Geometry check sheet. Reference: the model listing, model coordinates, mm. A direction names the side the tool comes from. Coordinates: 2 decimals unless noted, no trailing zeros. Loops run counter-clockwise (first coordinate to the right, second up) from the corner with the lowest first, then second, coordinate; pieces in that order, holes last.
from build123d import *

# Parameters (mm, degrees)
F1_DEPTH    = 10
F2_T1_DEPTH = 36.6968120455
F3_W        = 4.5079379342
F3_H        = 2.6771172415
F4_DEPTH    = 5
F6_D        = 1
F6_DEPTH    = 10
F6_TIP      = 0.3004303095


# Not quite as in the source:
# - a fillet or chamfer that OpenCascade refuses, or shapes differently, is made with other operations: its cross-section is extruded or revolved along the edge and cut away or added


with BuildPart() as f1:
    # F0 (on Top) → F1 (new body)
    with BuildSketch(Plane.XY):
        with BuildLine():
            ThreePointArc((0, -5), (-5, 0), (0, 5))
            Line((0, 5), (-10.5685128878, 5))
            Line((-10.5685128878, 5), (-10.5685128878, -5))
            Line((-10.5685128878, -5), (0, -5))
        make_face()
    extrude(amount=F1_DEPTH)

    # F2: chamfer of 5.08 on 2 edges, made by hand

    # F2_s2 → F2_t1 (cut)
    with BuildSketch(Plane.YZ.offset(-23.6326624666)):
        Polygon((-5, 4.92), (0.08, 10), (-5, 10), align=None)
        Polygon((5, 4.92), (-0.08, 10), (5, 10), align=None)
    extrude(amount=F2_T1_DEPTH, mode=Mode.SUBTRACT)

    # F3 (on face) → F4 (join)
    with BuildSketch(Plane(origin=(0, -4.96, 4.96), x_dir=(1, 0, 0), z_dir=(0, -0.7071067812, 0.7071067812))):
        with Locations((-7.4802257586, 3.3821087563)):
            Rectangle(F3_W, F3_H)
    extrude(amount=F4_DEPTH)

    # F6
    with Locations(Plane(origin=(0, -8.4955339059, 8.4955339059), x_dir=(1, 0, 0), z_dir=(0, -0.7071067812, 0.7071067812))):
        with Locations((-7.4782376178, 3.3632300328)):
            Hole(F6_D / 2, depth=F6_DEPTH)
            with Locations((0, 0, -(F6_DEPTH + F6_TIP / 2))):  # 118° drill point
                Cone(0, F6_D / 2, F6_TIP, mode=Mode.SUBTRACT)


solid = f1.part
(1) Sectioned sample at A-A on x = -4.75. Record the cut outline in (y, z), and give its area (3 significant figures).
Findings:
outline: (-5, 0) - (-1.56, 0) - (-1.56, 8.36) - (-5, 4.92) - close; (1.56, 0) - (5, 0) - (5, 4.92) - (1.56, 8.36) - close
area: 45.7 mm2
(2) Scan lines: L1, parallel to X at y = -4.25, z = 10.25; L2, parallel to Y at x = -6, z = 9.75; L3, parallel to Y at x = -7.25, z = 3. Record each from-to range of solid material in increasing order.
Findings:
L1: x = -9.73 to -5.23
L2: y = -6.86 to -3.07, -0.17 to 0.17
L3: y = -5 to 5
(3) Access from +Z, -Z, +X, -X, +Y, -Y to the whole of each face (thin tool, end or side, straight path). Record for faces 1 (the flat face through (-7.51, -5.26, 8.15)), 2 (the cylindrical face through (-5, 0, 4)), 3 (the flat face through (-5, -5, 2)), 4 (the flat face through (-5.226, -4, 9)), 5 (the flat face through (-9.734, -4, 9)).
Findings:
face 1: +X, -X, -Y
face 2: +Z, -Z, +X
face 3: -Z, +X, -X, -Y
face 4: +Z, +X, -Y
face 5: +Z, -X, -Y
(4) Draft check along Z on faces 6 (the cylindrical face through (-7.955, -2.426, 7.395)), 7 (the flat face through (-10.569, 0, 4)), 8 (the flat face through (-7.512, -3.365, 10.041)). Enter one of: +Z half, -Z half, draft (parallel to the pull), parting line (faces both ways), or undercut.
Findings:
face 6: undercut
face 7: draft
face 8: +Z half
(5) Sectioned sample at C-C on y = -4. State how many separate pieces and enclosed holes the cut face has, and give its area (3 significant figures).
Findings:
separate pieces: 2
enclosed holes: 1
area: 60.8 mm2
(6) Gauge pin test, flat ends, axial feed: pin 1 Ø1 at (x, y) = (-4, -4) entering from +Z; pin 2 Ø6 at (x, y) = (-5.5, -0.5) entering from +Z; pin 3 Ø5.5 at (x, z) = (-6, 3.5) entering from -Y. Record the tip position at first contact, or that the pin passes through.
Findings:
pin 1: stops at z = 6.42
pin 2: stops at z = 10.18
pin 3: stops at y = -5
(7) Sectioned sample at D-D on x = -9.5. Record the cut outline in (y, z) (3 decimals), and give its area (3 significant figures).
Findings:
outline: (-7.051, 9.941) - (-3.515, 6.405) - (-5, 4.92) - (-5, 0) - (5, 0) - (5, 4.92) - (0, 9.92) - (-1.622, 8.298) - (-5.158, 11.834) - close
area: 87.6 mm2
(8) Sectioned sample at B-B on z = 2. Record the cut outline in (x, y).
Findings:
outline: (-10.57, -5) - (0, -5) arc R5 cw to (0, 5) - (-10.57, 5) - close
